from build123d import *

# Parameters (mm, degrees)
SKETCH1_R           = 6
BOSS_EXTRUDE1_DEPTH = 8


with BuildPart() as part:
    # Sketch1 → Boss-Extrude1 (new body)
    with BuildSketch(Plane(origin=(0, 0, 0), x_dir=(1, 0, 0), z_dir=(0, 1, 0))):
        with BuildLine():
            Line((-25.10169054, -0.115674765), (-0.10169054, -0.115674765))
            Line((-0.10169054, -0.115674765), (-0.10169054, 29.884325235))
            ThreePointArc((-0.10169054, 29.884325235), (-3.030622728, 36.955393047), (-10.10169054, 39.884325235))
            Line((-10.10169054, 39.884325235), (-35.10169054, 39.884325235))
            Line((-35.10169054, 39.884325235), (-35.10169054, 19.884325235))
            Line((-35.10169054, 19.884325235), (-55.10169054, 19.884325235))
            Line((-55.10169054, 19.884325235), (-55.10169054, 39.884325235))
            Line((-55.10169054, 39.884325235), (-75.10169054, 39.884325235))
            ThreePointArc((-75.10169054, 39.884325235), (-82.172758352, 36.955393047), (-85.10169054, 29.884325235))
            Line((-85.10169054, 29.884325235), (-85.10169054, 10.884325235))
            ThreePointArc((-85.10169054, 10.884325235), (-64.10169054, -10.115674765), (-85.10169054, -31.115674765))
            Line((-85.10169054, -31.115674765), (-85.10169054, -50.115674765))
            ThreePointArc((-85.10169054, -50.115674765), (-82.172758352, -57.186742577), (-75.10169054, -60.115674765))
            Line((-75.10169054, -60.115674765), (-55.10169054, -60.115674765))
            Line((-55.10169054, -60.115674765), (-55.10169054, -40.115674765))
            Line((-55.10169054, -40.115674765), (-35.10169054, -40.115674765))
            Line((-35.10169054, -40.115674765), (-35.10169054, -60.115674765))
            Line((-35.10169054, -60.115674765), (-10.10169054, -60.115674765))
            ThreePointArc((-10.10169054, -60.115674765), (-3.030622728, -57.186742577), (-0.10169054, -50.115674765))
            Line((-0.10169054, -50.115674765), (-0.10169054, -20.115674765))
            Line((-0.10169054, -20.115674765), (-25.10169054, -20.115674765))
            ThreePointArc((-25.10169054, -20.115674765), (-35.10169054, -10.115674765), (-25.10169054, -0.115674765))
        make_face()
        with Locations((-15.10169054, 24.884325235)):
            Circle(SKETCH1_R, mode=Mode.SUBTRACT)
        with Locations((-15.10169054, -45.115674765)):
            Circle(SKETCH1_R, mode=Mode.SUBTRACT)
    extrude(amount=BOSS_EXTRUDE1_DEPTH)


solid = part.part
Geometry: final body of the model. Coordinates: model frame, mm. A direction names the side the tool comes from. Give positions to 0.01 mm unless a question says otherwise; leave off trailing zeros. Order: outer loops, then holes, each group sorted by start corner. A loop starts at its lowest first (then second) coordinate and runs counter-clockwise, first axis right, second up. Notation, with made-up numbers: (15, 27) - (34, 27) arc R25 cw to (34, 47) - close; hole circle Ø7 at (51, -17.75). An arc over 180 degrees is marked (long way). Use CSV: the item, a comma, the result in double quotes.
1. Section query A-A (x = -23). Output: boundary loops of the cut face in (y, z), plus the area to 3 significant figures.
Answers below:
outline,"(0, -39.88) - (8, -39.88) - (8, 0.12) - (0, 0.12) - close; (0, 20.12) - (8, 20.12) - (8, 60.12) - (0, 60.12) - close"
area,"640 mm2"
2. Section query D-D (x = -67). Output: boundary loops of the cut face in (y, z), plus the area to 3 significant figures.
Answers below:
outline,"(0, -39.88) - (8, -39.88) - (8, -0.53) - (0, -0.53) - close; (0, 20.76) - (8, 20.76) - (8, 60.12) - (0, 60.12) - close"
area,"630 mm2"
3. Material intervals for line 1 along Z through (x, y) = (-24.5, 1.5); line 2 along Z through (x, y) = (-14.5, 5); line 3 along Z through (x, y) = (-30, 3.25), sorted ascending. Write a range as from..to.
Answers below:
line 1,"-39.88..0.12, 20.12..60.12"
line 2,"-39.88..-30.85, -18.91..0.12, 20.12..39.15, 51.09..60.12"
line 3,"-39.88..1.4, 18.83..60.12"
4. Section query C-C (y = 6.25). Output: boundary loops of the cut face in (x, z).
Answers below:
outline,"(-85.1, -29.88) arc R10 ccw to (-75.1, -39.88) - (-55.1, -39.88) - (-55.1, -19.88) - (-35.1, -19.88) - (-35.1, -39.88) - (-10.1, -39.88) arc R10 ccw to (-0.1, -29.88) - (-0.1, 0.12) - (-25.1, 0.12) arc R10 cw to (-25.1, 20.12) - (-0.1, 20.12) - (-0.1, 50.12) arc R10 ccw to (-10.1, 60.12) - (-35.1, 60.12) - (-35.1, 40.12) - (-55.1, 40.12) - (-55.1, 60.12) - (-75.1, 60.12) arc R10 ccw to (-85.1, 50.12) - (-85.1, 31.12) arc R21 cw to (-85.1, -10.88) - close; hole circle Ø12 at (-15.1, -24.88); hole circle Ø12 at (-15.1, 45.12)"
5. Contact query for flat-ended pins moving along their axis: pin 1 (4 mm diameter, centred on x = -45.5, y = 4, fed in from +Z); pin 2 (4 mm diameter, centred on x = -46.5, y = 4, fed in from -Z). Output: stop coordinate, or through.
Answers below:
pin 1,"z = 40.12"
pin 2,"z = -19.88"
6. Access query for faces 4 (the face through (-45, 4, 40.116)), 5 (the face through (-55.102, 4, -30)), 6 (the face through (-21.096, 3.944, -25.148)). Directions: +Z, -Z, +X, -X, +Y, -Y. A direction counts if a zero-diameter tool reaches every point of the face in a straight line with its end or side. Return the directions, or none.
Answers below:
face 4,"+Z, +Y, -Y"
face 5,"-Z, +Y, -Y"
face 6,"+Y, -Y"
7. Section query B-B (z = 48). Output: boundary loops of the cut face in (x, y).
Answers below:
outline,"(-85.1, 0) - (-55.1, 0) - (-55.1, 8) - (-85.1, 8) - close; (-35.1, 0) - (-20.36, 0) - (-20.36, 8) - (-35.1, 8) - close; (-9.84, 0) - (-0.1, 0) - (-0.1, 8) - (-9.84, 8) - close"
8. Mould query, pull axis X, two halves, no side actions, for faces 1 (the face through (-82.25, 3.94, 57.11)), 2 (the face through (-22, 4, -39.884)), 3 (the face through (-19.524, 3.944, 41.061)). Classes: +X half, -X half, draft (parallel to the pull), parting line (faces both ways), or undercut.
Answers below:
face 1,"-X half"
face 2,"draft"
face 3,"undercut"
